Check sheet for the drawn part. Datum: minimum x, y, z corner. Units: mm. A direction names the side the tool comes from. Give positions to 0.01 mm unless a question says otherwise; leave off trailing zeros. Loops run counter-clockwise (first coordinate to the right, second up) from the corner with the lowest first, then second, coordinate; pieces in that order, holes last.
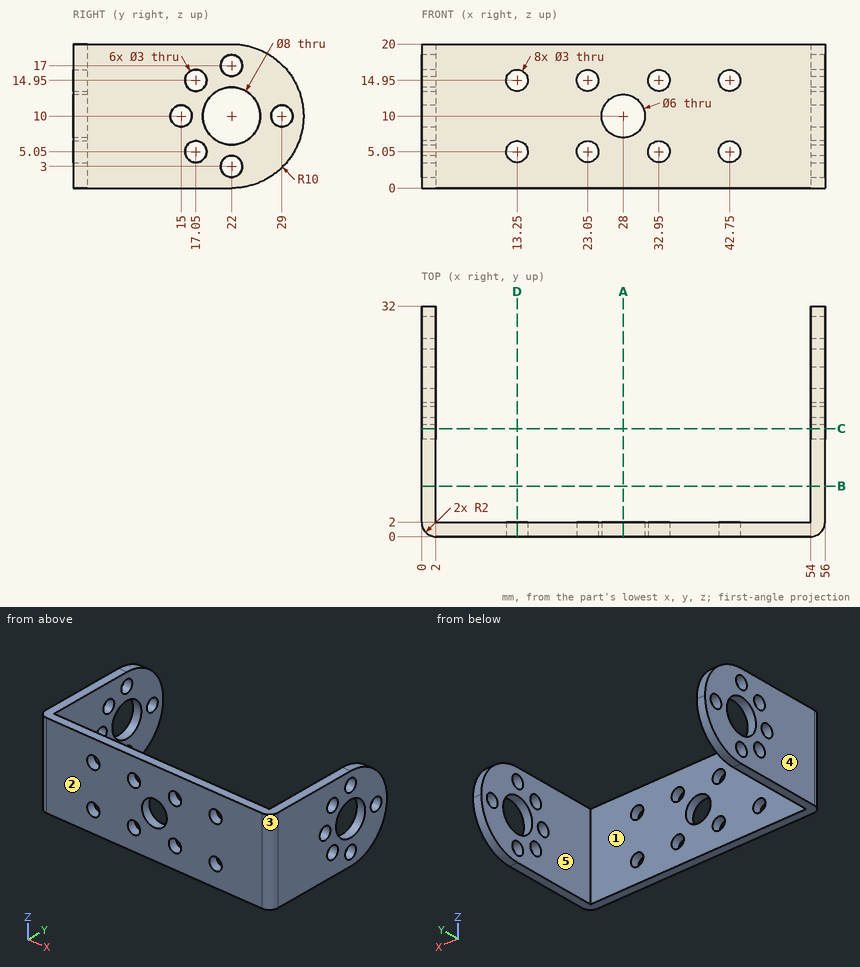
(1) Access from +Z, -Z, +X, -X, +Y, -Y to the whole of each face (thin tool, end or side, straight path). Record for the marked faces 4 and 5.
(2) Section check C-C on y = 15. Record the boundary of the cut face in (x, z), plus the area to 3 significant figures.
(3) Release check for a two-part mould opening along X. For the marked faces 1, 2 and 3 record: pulls with the +X half, pulls with the -X half, needs draft (parallel to the pull), parting line crosses it, or undercut.
(4) Section check D-D on x = 13.25. Record the boundary of the cut face in (y, z).
(5) Section check B-B on y = 7. Record the boundary of the cut face in (x, z), plus the area to 3 significant figures.
(6) Material ranges on line 1 (X direction, y = 22, z = 5); line 2 (Y direction, x = 40.5, z = 16.75); line 3 (Y direction, x = 1.55, z = 3), recorded low to high.
(7) Gauge pin test, flat end, axial feed: pin 1 Ø6 at (x, z) = (22.5, 11) entering from +Y. Record the tip position at first contact, or that the pin passes through.
(8) Section check A-A on x = 28. Record the boundary of the cut face in (y, z).
Computed values:
1. face 4: +Z, -Z, -X, +Y, -Y
1. face 5: +Z, -Z, +Y
2. outline: (0, 0) - (2, 0) - (2, 8.5) - (0, 8.5) - close; (0, 11.5) - (2, 11.5) - (2, 20) - (0, 20) - close; (54, 0) - (56, 0) - (56, 8.5) - (54, 8.5) - close; (54, 11.5) - (56, 11.5) - (56, 20) - (54, 20) - close
2. area: 68.0 mm2
3. face 1: undercut
3. face 2: needs draft
3. face 3: pulls with the +X half
4. outline: (0, 0) - (2, 0) - (2, 3.55) - (0, 3.55) - close; (0, 6.55) - (2, 6.55) - (2, 13.45) - (0, 13.45) - close; (0, 16.45) - (2, 16.45) - (2, 20) - (0, 20) - close
5. outline: (0, 0) - (2, 0) - (2, 20) - (0, 20) - close; (54, 0) - (56, 0) - (56, 20) - (54, 20) - close
5. area: 80.0 mm2
6. line 1: x = 0 to 2, 54 to 56
6. line 2: y = 0 to 2
6. line 3: y = 0.05 to 20.5, 23.5 to 29.14
7. pin 1: stops at y = 2
8. outline: (0, 0) - (2, 0) - (2, 7) - (0, 7) - close; (0, 13) - (2, 13) - (2, 20) - (0, 20) - close
